Work out the finished part from the listing and answer in its coordinate system (mm). Give positions to 0.01 mm unless a question says otherwise; leave off trailing zeros. Write each loop counter-clockwise with the first axis right and the second up, starting at its lowest first coordinate (ties: lowest second). Pieces come first, ordered by that corner, then holes. Notation, with made-up numbers: (-39, 69) -> (-7, 69) arc R17 cw to (-7, 99) -> close; hole circle Ø10 at (1, 65). An arc over 180 degrees is marked (long way). Use a Markdown table: item, result. Add a question column.
Q1. Section A-A, the plane x = -35 is taken. Give the vertices of the cut face in (y, z), plus the area to 3 significant figures.
Q2. Consider line 1 (Y direction, x = 36, z = 0.55); line 2 (Y direction, x = 111, z = 1.4); line 3 (X direction, y = -170.9, z = 1). Determine where each line is inside the solid, lowest interval first.
Q3. Section C-C, the plane x = 108.5 is taken. Give the vertices of the cut face in (y, z), plus the area to 3 significant figures.
Q4. Each of these flat-tipped pins is pushed along its axis until it touches: pin 1 Ø0.8 at (x, z) = (123.5, 0.5) entering from +Y; pin 2 Ø0.8 at (y, z) = (-179.5, 0.5) entering from +X; pin 3 Ø0.5 at (y, z) = (40, 1) entering from +X. Where does it stop, or does it pass through?
Q5. Section B-B, the plane z = 0.55 is taken. State how many separate pieces and enclosed holes the cut face has, plus the area to 3 significant figures.
from build123d import *

# Parameters (mm, degrees)
SKETCH_1_R      = 1.5
SKETCH_1_R_2    = 1
SKETCH_1_R_3    = 6.6
SKETCH_1_R_4    = 1.55
EXTRUDE_1_DEPTH = 1.6


with BuildPart() as part:
    # 草图1 → 凸台-拉伸1 (new body)
    with BuildSketch(Plane.XY):
        with BuildLine():
            Line((28.3, -182.6), (21.7, -182.6))
            ThreePointArc((21.7, -182.6), (20.285786438, -182.014213562), (19.7, -180.6))
            Line((19.7, -180.6), (19.7, -172.540561017))
            ThreePointArc((19.7, -172.540561017), (15.702142896, -161.229504731), (5.484445076, -154.942891414))
            Line((5.484445076, -154.942891414), (-60.051234743, -140.849196829))
            ThreePointArc((-60.051234743, -140.849196829), (-62.889484138, -139.102915353), (-64, -135.960955273))
            Line((-64, -135.960955273), (-64, -103))
            ThreePointArc((-64, -103), (-62.535533906, -99.464466094), (-59, -98))
            Line((-59, -98), (-43.626727815, -98))
            ThreePointArc((-43.626727815, -98), (-23.924293673, -90.623308531), (-13.911111388, -72.120939259))
            Line((-13.911111388, -72.120939259), (-10.843078735, -49.997710609))
            ThreePointArc((-10.843078735, -49.997710609), (-10.045683656, -45.018963187), (-9.039840064, -40.078108658))
            Line((-9.039840064, -40.078108658), (-1.124995937, -4.987666714))
            ThreePointArc((-1.124995937, -4.987666714), (0.57285044, -0.292525766), (3.380699046, 3.835793148))
            Line((3.380699046, 3.835793148), (21.00417619, 23.831661447))
            ThreePointArc((21.00417619, 23.831661447), (24.709403034, 29.987566958), (26, 37.05568114))
            Line((26, 37.05568114), (26, 42))
            Line((26, 42), (46, 42))
            Line((46, 42), (46, 37.05568114))
            ThreePointArc((46, 37.05568114), (47.290596966, 29.987566958), (50.99582381, 23.831661447))
            Line((50.99582381, 23.831661447), (68.619300954, 3.835793148))
            ThreePointArc((68.619300954, 3.835793148), (71.42714956, -0.292525766), (73.124995937, -4.987666714))
            Line((73.124995937, -4.987666714), (81.039840064, -40.078108658))
            ThreePointArc((81.039840064, -40.078108658), (82.045683656, -45.018963187), (82.843078735, -49.997710609))
            Line((82.843078735, -49.997710609), (85.911111388, -72.120939259))
            ThreePointArc((85.911111388, -72.120939259), (95.924293673, -90.623308531), (115.626727815, -98))
            Line((115.626727815, -98), (131, -98))
            ThreePointArc((131, -98), (134.535533906, -99.464466094), (136, -103))
            Line((136, -103), (136, -135.960955273))
            ThreePointArc((136, -135.960955273), (134.889484138, -139.102915353), (132.051234743, -140.849196829))
            Line((132.051234743, -140.849196829), (66.515554924, -154.942891414))
            ThreePointArc((66.515554924, -154.942891414), (56.297857104, -161.229504731), (52.3, -172.540561017))
            Line((52.3, -172.540561017), (52.3, -180.6))
            ThreePointArc((52.3, -180.6), (51.714213562, -182.014213562), (50.3, -182.6))
            Line((50.3, -182.6), (43.7, -182.6))
            ThreePointArc((43.7, -182.6), (42.285786438, -182.014213562), (41.7, -180.6))
            Line((41.7, -180.6), (41.7, -178.737691249))
            ThreePointArc((41.7, -178.737691249), (42.017498822, -172.573354043), (42.966635106, -166.474255831))
            Line((42.966635106, -166.474255831), (47.982301372, -142.452687084))
            ThreePointArc((47.982301372, -142.452687084), (45.547777581, -132.431388668), (36.235628393, -128))
            Line((36.235628393, -128), (35.764371607, -128))
            ThreePointArc((35.764371607, -128), (26.452222419, -132.431388668), (24.017698628, -142.452687084))
            Line((24.017698628, -142.452687084), (29.033364894, -166.474255831))
            ThreePointArc((29.033364894, -166.474255831), (29.982501178, -172.573354043), (30.3, -178.737691249))
            Line((30.3, -178.737691249), (30.3, -180.6))
            ThreePointArc((30.3, -180.6), (29.714213562, -182.014213562), (28.3, -182.6))
        make_face()
        with Locations((2, -12.95)):
            Circle(SKETCH_1_R, mode=Mode.SUBTRACT)
        with Locations(Location((70, -12.95, 0), (0, 0, 180))):
            Circle(SKETCH_1_R, mode=Mode.SUBTRACT)
        with Locations((-5.6215, -80.046)):
            Circle(SKETCH_1_R, mode=Mode.SUBTRACT)
        with Locations(Location((77.6215, -80.046, 0), (0, 0, 180))):
            Circle(SKETCH_1_R, mode=Mode.SUBTRACT)
        with Locations((25.3, -170.9)):
            Circle(SKETCH_1_R_2, mode=Mode.SUBTRACT)
        with Locations((25.3, -181.1)):
            Circle(SKETCH_1_R_2, mode=Mode.SUBTRACT)
        with Locations((21.2, -176)):
            Circle(SKETCH_1_R_2, mode=Mode.SUBTRACT)
        with Locations(Location((46.7, -181.1, 0), (0, 0, 180))):
            Circle(SKETCH_1_R_2, mode=Mode.SUBTRACT)
        with Locations(Location((50.8, -176, 0), (0, 0, 180))):
            Circle(SKETCH_1_R_2, mode=Mode.SUBTRACT)
        with Locations(Location((46.7, -170.9, 0), (0, 0, 180))):
            Circle(SKETCH_1_R_2, mode=Mode.SUBTRACT)
        with Locations((28, 39)):
            Circle(SKETCH_1_R_2, mode=Mode.SUBTRACT)
        with Locations(Location((44, 39, 0), (0, 0, 180))):
            Circle(SKETCH_1_R_2, mode=Mode.SUBTRACT)
        with Locations((44, 20)):
            Circle(SKETCH_1_R_2, mode=Mode.SUBTRACT)
        with Locations(Location((28, 20, 0), (0, 0, 180))):
            Circle(SKETCH_1_R_2, mode=Mode.SUBTRACT)
        with Locations((36, 8)):
            Circle(SKETCH_1_R_3, mode=Mode.SUBTRACT)
        with Locations((-59, -103)):
            Circle(SKETCH_1_R_4, mode=Mode.SUBTRACT)
        with Locations((-59, -135.960955273)):
            Circle(SKETCH_1_R_4, mode=Mode.SUBTRACT)
        with Locations(Location((-51, -135.960955273, 0), (0, 0, 180))):
            Circle(SKETCH_1_R_4, mode=Mode.SUBTRACT)
        with Locations(Location((-51, -103, 0), (0, 0, 180))):
            Circle(SKETCH_1_R_4, mode=Mode.SUBTRACT)
        with Locations(Location((131, -135.960955273, 0), (0, 0, 180))):
            Circle(SKETCH_1_R_4, mode=Mode.SUBTRACT)
        with Locations((123, -135.960955273)):
            Circle(SKETCH_1_R_4, mode=Mode.SUBTRACT)
        with Locations((123, -103)):
            Circle(SKETCH_1_R_4, mode=Mode.SUBTRACT)
        with Locations(Location((131, -103, 0), (0, 0, 180))):
            Circle(SKETCH_1_R_4, mode=Mode.SUBTRACT)
        with BuildLine():
            Line((11, -80.046), (11, -45))
            ThreePointArc((11, -45), (36, -20), (61, -45))
            Line((61, -45), (61, -80.046))
            ThreePointArc((61, -80.046), (36, -105.046), (11, -80.046))
        make_face(mode=Mode.SUBTRACT)
        with BuildLine():
            Line((-44, -111.880477636), (-24, -111.880477636))
            ThreePointArc((-24, -111.880477636), (-22.4, -113.480477636), (-24, -115.080477636))
            Line((-24, -115.080477636), (-44, -115.080477636))
            ThreePointArc((-44, -115.080477636), (-45.6, -113.480477636), (-44, -111.880477636))
        make_face(mode=Mode.SUBTRACT)
        with BuildLine():
            Line((-44, -127.080477636), (-24, -127.080477636))
            ThreePointArc((-24, -127.080477636), (-22.4, -125.480477636), (-24, -123.880477636))
            Line((-24, -123.880477636), (-44, -123.880477636))
            ThreePointArc((-44, -123.880477636), (-45.6, -125.480477636), (-44, -127.080477636))
        make_face(mode=Mode.SUBTRACT)
        with BuildLine():
            Line((116, -111.880477636), (96, -111.880477636))
            ThreePointArc((96, -111.880477636), (94.4, -113.480477636), (96, -115.080477636))
            Line((96, -115.080477636), (116, -115.080477636))
            ThreePointArc((116, -115.080477636), (117.6, -113.480477636), (116, -111.880477636))
        make_face(mode=Mode.SUBTRACT)
        with BuildLine():
            Line((116, -127.080477636), (96, -127.080477636))
            ThreePointArc((96, -127.080477636), (94.4, -125.480477636), (96, -123.880477636))
            Line((96, -123.880477636), (116, -123.880477636))
            ThreePointArc((116, -123.880477636), (117.6, -125.480477636), (116, -127.080477636))
        make_face(mode=Mode.SUBTRACT)
    extrude(amount=EXTRUDE_1_DEPTH)


solid = part.part
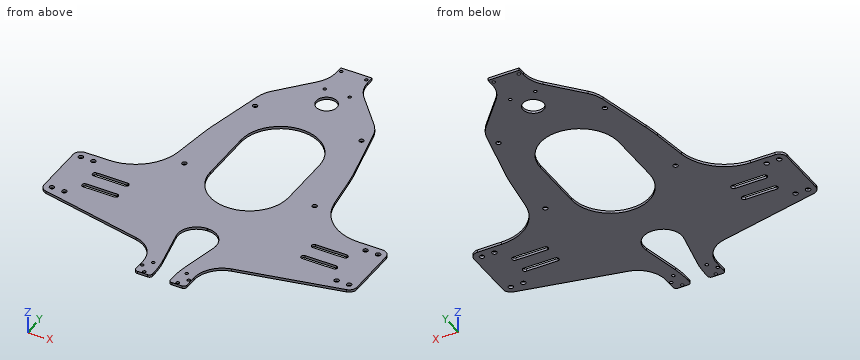
Result set:
| question | item | result |
|---|---|---|
| 1 | outline | (-146.24, 0) -> (-127.08, 0) -> (-127.08, 1.6) -> (-146.24, 1.6) -> close; (-123.88, 0) -> (-115.08, 0) -> (-115.08, 1.6) -> (-123.88, 1.6) -> close; (-111.88, 0) -> (-96.73, 0) -> (-96.73, 1.6) -> (-111.88, 1.6) -> close |
| 1 | area | 69.0 mm2 |
| 2 | line 1 | y = -128 to -105.05, -20 to 1.4, 14.6 to 42 |
| 2 | line 2 | y = -145.38 to -127.08, -123.88 to -115.08, -111.88 to -97.64 |
| 2 | line 3 | x = 19.63 to 24.3, 26.3 to 29.79, 42.21 to 45.7, 47.7 to 52.37 |
| 3 | outline | (-145.91, 0) -> (-127.08, 0) -> (-127.08, 1.6) -> (-145.91, 1.6) -> close; (-123.88, 0) -> (-115.08, 0) -> (-115.08, 1.6) -> (-123.88, 1.6) -> close; (-111.88, 0) -> (-97.14, 0) -> (-97.14, 1.6) -> (-111.88, 1.6) -> close |
| 3 | area | 67.8 mm2 |
| 4 | pin 1 | stops at y = -98 |
| 4 | pin 2 | stops at x = 52.3 |
| 4 | pin 3 | stops at x = 46 |
| 5 | separate pieces | 1 |
| 5 | enclosed holes | 28 |
| 5 | area | 17,000 mm2 |
